The model under review builds one solid part; all positions refer to its coordinate system, in mm. A direction names the side the tool comes from. Give positions to 0.01 mm unless a question says otherwise; leave off trailing zeros. Order: outer loops, then holes, each group sorted by start corner. A loop starts at its lowest first (then second) coordinate and runs counter-clockwise, first axis right, second up. Notation, with made-up numbers: (-3.75, 57.5) - (31.25, 57.5) arc R19 ccw to (31.25, 84.5) - close; hole circle Ø8 at (53.25, -24.5). An arc over 180 degrees is marked (long way). Use CSV: the item, a comma, the result in double quotes. Start each with the question number.
1. For pin 1 (3 mm diameter, centred on y = 32, z = 3, fed in from +X); pin 2 (3 mm diameter, centred on x = 13.5, y = 7.5, fed in from +Z); pin 3 (2 mm diameter, centred on x = 19, z = -1, fed in from -Y), all flat-tipped, find the tip position at first contact; note any pin that passes through.
2. Take a section at C-C, the plane z = 8.25. State the section outline as (x, y) points.
3. Take a section at B-B, the plane x = 2. State the section outline as (y, z) points, then the cut area to 3 significant figures.
4. Take a section at D-D, the plane x = -13.5. State the section outline as (y, z) points.
5. To check wall thickness, follow line 1 (Y direction, x = 2, z = -0.45); line 2 (Y direction, x = -15, z = 8); line 3 (X direction, y = -2.5, z = -1.5). State the ranges of each line that lie inside material, in increasing order. Write a range as [from, to].
6. Machinability: for faces 1 (the flat face through (16.5, 32, 4)), 2 (the flat face through (-20, -30, 0)), 3 (the flat face through (-20, 30, 0)), 4 (the flat face through (19, -30, 0)), which of the approach directions +Z, -Z, +X, -X, +Y, -Y give a long, thin tool a straight path to every point of the face, cutting with its end or side? Answer none if there is none.
7. Draft analysis for pull direction Y (two halves, no side actions). For faces 5 (the flat face through (0, 34, 4)), 6 (the flat face through (0, -32, 11)), 7 (the flat face through (0, -30, 6)), state which applies: released by +Y, released by -Y, zero draft, split by the parting line, or undercut.
8. Take a section at A-A, the plane y = -3. State the section outline as (x, z) points, then the cut area to 3 significant figures.
```python
from build123d import *

# Parameters (mm, degrees)
SKETCH1_W           = 45
SKETCH1_H           = 60
SKETCH1_R           = 10
BOSS_EXTRUDE1_DEPTH = 2
SKETCH3_W           = 33
SKETCH3_H           = 4
BOSS_EXTRUDE3_DEPTH = 13


with BuildPart() as part:
    # Sketch1 → Boss-Extrude1 (new, symmetric)
    with BuildSketch(Plane.XY):
        Rectangle(SKETCH1_W, SKETCH1_H)
        with Locations((2, -3)):
            Circle(SKETCH1_R, mode=Mode.SUBTRACT)
    extrude(amount=BOSS_EXTRUDE1_DEPTH, both=True)

    # Sketch3 → Boss-Extrude3 (add)
    with BuildSketch(Plane(origin=(0, 0, -2), x_dir=(-1, 0, 0), z_dir=(0, 0, -1))):
        with Locations((0, 32)):
            Rectangle(SKETCH3_W, SKETCH3_H)
        with Locations((0, -32)):
            Rectangle(SKETCH3_W, SKETCH3_H)
    extrude(amount=-BOSS_EXTRUDE3_DEPTH)


solid = part.part
```
Determined:
1,pin 1,"stops at x = 16.5"
1,pin 2,"stops at z = 2"
1,pin 3,"stops at y = -30"
2,outline,"(-16.5, -34) - (16.5, -34) - (16.5, -30) - (-16.5, -30) - close; (-16.5, 30) - (16.5, 30) - (16.5, 34) - (-16.5, 34) - close"
3,outline,"(-34, -2) - (-13, -2) - (-13, 2) - (-30, 2) - (-30, 11) - (-34, 11) - close; (7, -2) - (34, -2) - (34, 11) - (30, 11) - (30, 2) - (7, 2) - close"
3,area,"264 mm²"
4,outline,"(-34, -2) - (34, -2) - (34, 11) - (30, 11) - (30, 2) - (-30, 2) - (-30, 11) - (-34, 11) - close"
5,line 1,"y = [-34, -13], [7, 34]"
5,line 2,"y = [-34, -30], [30, 34]"
5,line 3,"x = [-22.5, -7.99], [11.99, 22.5]"
6,face 1,"+Z, -Z, +X, +Y"
6,face 2,"+Z, -Z, -X, -Y"
6,face 3,"+Z, -Z, -X, +Y"
6,face 4,"+Z, -Z, +X, -Y"
7,face 5,"released by +Y"
7,face 6,"zero draft"
7,face 7,"undercut"
8,outline,"(-22.5, -2) - (-8, -2) - (-8, 2) - (-22.5, 2) - close; (12, -2) - (22.5, -2) - (22.5, 2) - (12, 2) - close"
8,area,"100 mm²"
